Geometry check sheet. Reference: the model listing, model coordinates, mm. Face numbers are marked on the shaded views. A direction names the side the tool comes from. Round coordinates to 2 decimals unless told otherwise and drop trailing zeros. Order: outer loops, then holes, each group sorted by start corner. A loop starts at its lowest first (then second) coordinate and runs counter-clockwise, first axis right, second up.
(1) Sectioned sample at C-C (z = 0). Record the boundary of the cut face in (x, y) (3 decimals).
(2) Sectioned sample at B-B (y = 4.75). Record the boundary of the cut face in (x, z) (3 decimals).
(3) Material ranges on line 1 along Z through (x, y) = (8, 0.9); line 2 along X through (y, z) = (8.25, -4.25) (3 decimals), recorded low to high.
(4) Release check for a two-part mould opening along Z. For the marked faces 1, 2 and 3 record: +Z half, -Z half, draft (parallel to the pull), parting line (faces both ways), or undercut.
(5) Go/stop test with a flat-tipped pin: pin 1 (4 mm diameter, centred on x = 8, z = 0, fed in from +Y) (3 decimals). Record where the tip stops, or that it passes through.
(6) Set-up check for the marked faces 4 and 5: record each of +Z, -Z, +X, -X, +Y, -Y from which the full face is reachable in a straight line by a thin tool's end or side.
(7) Sectioned sample at D-D (z = 8). Record the boundary of the cut face in (x, y) (3 decimals), plus the area to 3 significant figures.
(8) Sectioned sample at A-A (x = 0). Record the boundary of the cut face in (y, z) (3 decimals), plus the area to 3 significant figures.
from build123d import *

# Parameters (mm, degrees)
SKETCH1_W                 = 28
SKETCH1_H                 = 28
BOSS_EXTRUDE1_DEPTH       = 3.175
SKETCH2_R                 = 5
CUT_EXTRUDE1_DEPTH        = 21.05194816
F_3_0MM_DOWEL_HOLE1_D     = 3.3
F_3_0MM_DOWEL_HOLE1_DEPTH = 15
F_3_0MM_DOWEL_HOLE1_TIP   = 0.991420021
BOSS_EXTRUDE3_DEPTH       = 6
CIRPATTERN2_COUNT         = 4
CHAMFER2_SIZE             = 0.5


with BuildPart() as part:
    # Sketch1 → Boss-Extrude1 (new body)
    with BuildSketch(Plane(origin=(0, 0, 0), x_dir=(1, 0, 0), z_dir=(0, 1, 0))):
        Rectangle(SKETCH1_W, SKETCH1_H)
    extrude(amount=BOSS_EXTRUDE1_DEPTH)

    # Sketch2 → Cut-Extrude1 (cut, through all)
    with BuildSketch(Plane(origin=(0, 3.175, 0), x_dir=(1, 0, 0), z_dir=(0, 1, 0))):
        with Locations(Location((0, 0, 0), (0, 0, 270))):
            Circle(SKETCH2_R)
    extrude(amount=-CUT_EXTRUDE1_DEPTH, mode=Mode.SUBTRACT)

    # Ø3.0mm Dowel Hole1
    with Locations(Plane(origin=(0, 3.175, 0), x_dir=(1, 0, 0), z_dir=(0, 1, 0))):
        with Locations((8, 0), (0, -8), (-8, 0), (0, 8)):
            Hole(F_3_0MM_DOWEL_HOLE1_D / 2, depth=F_3_0MM_DOWEL_HOLE1_DEPTH)
            with Locations((0, 0, -(F_3_0MM_DOWEL_HOLE1_DEPTH + F_3_0MM_DOWEL_HOLE1_TIP / 2))):  # 118° drill point
                Cone(0, F_3_0MM_DOWEL_HOLE1_D / 2, F_3_0MM_DOWEL_HOLE1_TIP, mode=Mode.SUBTRACT)

    # Sketch7 → Boss-Extrude3 (add)
    with BuildSketch(Plane(origin=(0, 3.175, 0), x_dir=(1, 0, 0), z_dir=(0, 1, 0))):
        Polygon((-13.75, -14), (13.75, -14), (9.966182344, -10.825), (-9.966182344, -10.825), align=None)
    boss_extrude3 = extrude(amount=BOSS_EXTRUDE3_DEPTH)

    # CirPattern2: Boss-Extrude3 ×4 about axis
    cirpattern2_axis = Axis((0, 0, 0), (0, 1, 0))
    for i in range(1, CIRPATTERN2_COUNT):
        add(boss_extrude3.rotate(cirpattern2_axis, i * 360 / CIRPATTERN2_COUNT))

    # Chamfer2
    chamfer2_edges = [part.edges().sort_by_distance(p)[0] for p in [
        (0, 3.175, 10.825),
        (10.825, 3.175, 0),
        (0, 3.175, -10.825),
        (-10.825, 3.175, 0),
    ]]
    chamfer(chamfer2_edges, length=CHAMFER2_SIZE)


solid = part.part
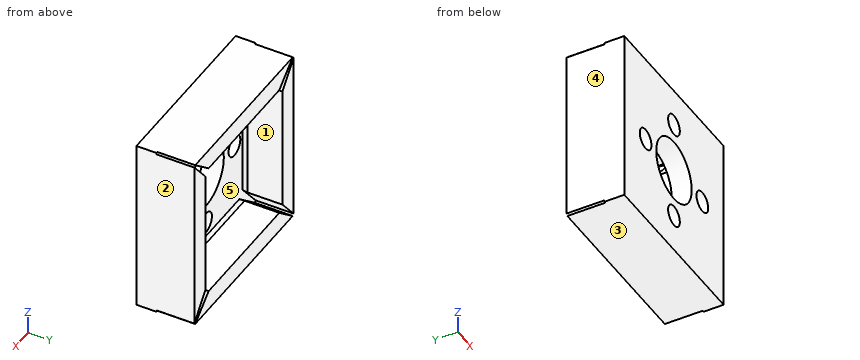
Answer below:
1. outline: (-14, 0) - (-9.65, 0) - (-9.65, 3.175) - (-10.325, 3.175) - (-10.825, 3.675) - (-10.825, 9.175) - (-14, 9.175) - close; (-6.35, 0) - (-5, 0) - (-5, 3.175) - (-6.35, 3.175) - close; (5, 0) - (6.35, 0) - (6.35, 3.175) - (5, 3.175) - close; (9.65, 0) - (14, 0) - (14, 9.175) - (10.825, 9.175) - (10.825, 3.675) - (10.325, 3.175) - (9.65, 3.175) - close
2. outline: (-14, -13.75) - (-10.825, -9.966) - (-10.825, 9.966) - (-14, 13.75) - close; (-13.75, -14) - (13.75, -14) - (9.966, -10.825) - (-9.966, -10.825) - close; (-13.75, 14) - (-9.966, 10.825) - (9.966, 10.825) - (13.75, 14) - close; (10.825, -9.966) - (14, -13.75) - (14, 13.75) - (10.825, 9.966) - close
3. line 1: z = -14 to -1.65, 1.65 to 14
3. line 2: x = -14 to -10.825, 10.825 to 14
4. face 1: undercut
4. face 2: draft
4. face 3: -Z half
5. pin 1: stops at y = 3.175
6. face 4: +Z, -Z, -X, +Y, -Y
6. face 5: +Y
7. outline: (-14, 0) - (-1.65, 0) - (-1.65, 3.175) - (-10.325, 3.175) - (-10.825, 3.675) - (-10.825, 9.175) - (-14, 9.175) - close; (1.65, 0) - (14, 0) - (14, 9.175) - (10.825, 9.175) - (10.825, 3.675) - (10.325, 3.175) - (1.65, 3.175) - close
7. area: 117 mm2
8. outline: (0, -14) - (9.175, -14) - (9.175, -10.825) - (3.675, -10.825) - (3.175, -10.325) - (3.175, -9.65) - (0, -9.65) - close; (0, -6.35) - (3.175, -6.35) - (3.175, -5) - (0, -5) - close; (0, 5) - (3.175, 5) - (3.175, 6.35) - (0, 6.35) - close; (0, 9.65) - (3.175, 9.65) - (3.175, 10.325) - (3.675, 10.825) - (9.175, 10.825) - (9.175, 14) - (0, 14) - close
8. area: 74.5 mm2
